```python
from build123d import *

# Parameters (mm, degrees)
SKETCH1_W           = 20
SKETCH1_H           = 155
BOSS_EXTRUDE1_DEPTH = 4
SKETCH2_W           = 20
SKETCH2_H           = 4
BOSS_EXTRUDE3_DEPTH = 50
RIB2_REACH          = 96.986
SKETCH7_WALL_W      = 290.205463948
SKETCH7_WALL_H      = 4
SKETCH8_W           = 20
SKETCH8_H           = 3
BOSS_EXTRUDE4_DEPTH = 3.5
SKETCH9_W           = 70
SKETCH9_H           = 5
BOSS_EXTRUDE6_DEPTH = 3
SKETCH10_W          = 10
SKETCH10_H          = 4
BOSS_EXTRUDE7_DEPTH = 8
SKETCH12_R          = 1.75
CUT_EXTRUDE1_DEPTH  = 10
SKETCH13_W          = 111.319070758
SKETCH13_H          = 99.743885808
CUT_EXTRUDE2_DEPTH  = 152
SKETCH14_W          = 50
SKETCH14_H          = 3
BOSS_EXTRUDE8_DEPTH = 6.5
FILLET1_R           = 1
FILLET2_R           = 2.5
SKETCH15_R          = 3.25
BOSS_EXTRUDE9_DEPTH = 3
FILLET3_R           = 10


with BuildPart() as part:
    # Sketch1 → Boss-Extrude1 (new body)
    with BuildSketch(Plane.XY):
        Rectangle(SKETCH1_W, SKETCH1_H)
    extrude(amount=BOSS_EXTRUDE1_DEPTH)

    # Sketch2 → Boss-Extrude3 (add)
    with BuildSketch(Plane.XY.offset(4)):
        with Locations((0, -75.5)):
            Rectangle(SKETCH2_W, SKETCH2_H)
    extrude(amount=BOSS_EXTRUDE3_DEPTH)

    # Sketch7 wall → Rib2 (add, up to next)
    with BuildSketch(Plane(origin=(0, -26, 16.5), x_dir=(0, 0.967074537263, -0.25449329928), z_dir=(0, 0.25449329928, 0.967074537263)), mode=Mode.PRIVATE) as rib2_sk1:
        Rectangle(SKETCH7_WALL_W, SKETCH7_WALL_H)
    rib2_tool1 = extrude(rib2_sk1.sketch, amount=-RIB2_REACH, mode=Mode.PRIVATE) - part.part
    add(rib2_tool1.solids().sort_by_distance((0, -26, 16.5))[0])

    # Sketch8 → Boss-Extrude4 (add)
    with BuildSketch(Plane.XY.offset(4)):
        with Locations((0, 76)):
            Rectangle(SKETCH8_W, SKETCH8_H)
    extrude(amount=BOSS_EXTRUDE4_DEPTH)

    # Sketch9 → Boss-Extrude6 (add)
    with BuildSketch(Plane.XY.offset(7.5)):
        with Locations((0, 77)):
            Rectangle(SKETCH9_W, SKETCH9_H)
    boss_extrude6 = extrude(amount=BOSS_EXTRUDE6_DEPTH)

    # Sketch10 → Boss-Extrude7 (add)
    with BuildSketch(Plane(origin=(0, 0, 7.5), x_dir=(-1, 0, 0), z_dir=(0, 0, -1))):
        with Locations((30, 76.5)):
            Rectangle(SKETCH10_W, SKETCH10_H)
        with Locations((-30, 76.5)):
            Rectangle(SKETCH10_W, SKETCH10_H)
    extrude(amount=BOSS_EXTRUDE7_DEPTH)

    # Sketch12 → Cut-Extrude1 (cut)
    with BuildSketch(Plane(origin=(0, 78.5, 0), x_dir=(1, 0, 0), z_dir=(0, 1, 0))):
        with Locations(Location((-31, -3, 0), (0, 0, 270))):
            Circle(SKETCH12_R)
        with Locations(Location((31, -3, 0), (0, 0, 270))):
            Circle(SKETCH12_R)
    extrude(amount=-CUT_EXTRUDE1_DEPTH, mode=Mode.SUBTRACT)

    # Sketch13 → Cut-Extrude2 (cut)
    with BuildSketch(Plane.XZ.offset(77.5)):
        with Locations((2.652852139, 20.474703111)):
            Rectangle(SKETCH13_W, SKETCH13_H)
    extrude(amount=-CUT_EXTRUDE2_DEPTH, mode=Mode.SUBTRACT)

    # Sketch14 → Boss-Extrude8 (add)
    with BuildSketch(Plane(origin=(0, 79.5, 0), x_dir=(1, 0, 0), z_dir=(0, 1, 0))):
        with Locations((0, -9)):
            Rectangle(SKETCH14_W, SKETCH14_H)
    boss_extrude8 = extrude(amount=BOSS_EXTRUDE8_DEPTH)

    # Mirror1: Boss-Extrude6, Boss-Extrude8 across plane
    add(boss_extrude6.mirror(Plane(origin=(0, 76, 0), x_dir=(0, 0, 1), z_dir=(0, -1, 0))))
    add(boss_extrude8.mirror(Plane(origin=(0, 76, 0), x_dir=(0, 0, 1), z_dir=(0, -1, 0))))

    # Fillet1
    fillet1_edges = [part.edges().sort_by_distance(p)[0] for p in [
        (30, 78.5, 7.5),
        (-30, 78.5, 7.5),
        (10, 76, 7.5),
        (-10, 76, 7.5),
        (0, 77.5, 7.5),
        (25, 76.5, 7.5),
        (-25, 76.5, 7.5),
    ]]
    fillet(fillet1_edges, radius=FILLET1_R - 0.0001)  # a hair under: the kernel refuses the full size

    # Fillet2
    fillet2_edges = [part.edges().sort_by_distance(p)[0] for p in [
        (-25, 79.5, 9),
        (25, 79.5, 9),
        (-25, 66, 9),
        (25, 66, 9),
        (-25, 72.5, 9),
        (25, 72.5, 9),
    ]]
    fillet(fillet2_edges, radius=FILLET2_R)

    # Sketch15 → Boss-Extrude9 (add)
    with BuildSketch(Plane(origin=(0, 0, 7.5), x_dir=(-1, 0, 0), z_dir=(0, 0, -1))):
        with BuildLine():
            Line((25, 86), (-25, 86))
            ThreePointArc((-25, 86), (0, 103.502), (25, 86))
        make_face()
        with Locations((0, 91.001)):
            Circle(SKETCH15_R, mode=Mode.SUBTRACT)
    extrude(amount=-BOSS_EXTRUDE9_DEPTH)

    # Fillet3
    fillet3_edges = [part.edges().sort_by_distance(p)[0] for p in [
        (-25, 86, 9),
        (25, 86, 9),
    ]]
    fillet(fillet3_edges, radius=FILLET3_R)


solid = part.part
```
The model under review builds one solid part; all positions refer to its coordinate system, in mm. A direction names the side the tool comes from. Round coordinates to 2 decimals unless told otherwise and drop trailing zeros. Order: outer loops, then holes, each group sorted by start corner. A loop starts at its lowest first (then second) coordinate and runs counter-clockwise, first axis right, second up. Notation, with made-up numbers: (48, -18.5) -> (76, -18.5) arc R25 cw to (76, 1.5) -> close; hole circle Ø8 at (48.5, -27.5). An arc over 180 degrees is marked (long way). Use a Markdown table: item, result.
Q1. We need section A-A on x = 0. Write out the cut boundary in (y, z), then the cut area to 3 significant figures.
Values:
| item | result |
|---|---|
| outline | (66, 7.5) -> (74.5, 7.5) -> (74.5, 0) -> (77.5, 0) -> (77.5, 6.5) arc R1 cw to (78.5, 7.5) -> (87.75, 7.5) -> (87.75, 10.5) -> (66, 10.5) -> close; (94.25, 7.5) -> (103.5, 7.5) -> (103.5, 10.5) -> (94.25, 10.5) -> close |
| area | 116 mm^2 |
Q2. We need section D-D on z = 9.5. Write out the cut boundary in (x, y).
Values:
| item | result |
|---|---|
| outline | (-35, 72.5) -> (-27.5, 72.5) arc R2.5 cw to (-25, 70) -> (-25, 68.5) arc R2.5 ccw to (-22.5, 66) -> (22.5, 66) arc R2.5 ccw to (25, 68.5) -> (25, 70) arc R2.5 cw to (27.5, 72.5) -> (35, 72.5) -> (35, 79.5) -> (27.5, 79.5) arc R2.5 cw to (25, 82) -> (25, 84.02) arc R10 ccw to (24.03, 88.31) arc R26.61 ccw to (-24.03, 88.31) arc R10 ccw to (-25, 84.02) -> (-25, 82) arc R2.5 cw to (-27.5, 79.5) -> (-35, 79.5) -> close; hole circle Ø6.5 at (0, 91) |
Q3. Clearance check with flat-ended pins moving along their axes: P1, Ø3.5, axis at x = -31.5, z = 9.5, coming from the +Y side; P2, Ø5, axis at x = -5, y = 79.5, coming from the -Z side; P3, Ø1.2, axis at y = 69, z = 9.5, coming from the -X side. State where each tip first meets the part, or that it passes through.
Values:
| item | result |
|---|---|
| P1 | stops at y = 79.5 |
| P2 | stops at z = 0 |
| P3 | stops at x = -25 |
Q4. We need section B-B on z = 3. Write out the cut boundary in (x, y), then the cut area to 3 significant figures.
Values:
| item | result |
|---|---|
| outline | (-35, 74.5) -> (-32.75, 74.5) -> (-32.75, 78.5) -> (-35, 78.5) -> close; (-29.25, 74.5) -> (-25, 74.5) -> (-25, 78.5) -> (-29.25, 78.5) -> close; (-10, 74.5) -> (10, 74.5) -> (10, 77.5) -> (-10, 77.5) -> close; (25, 74.5) -> (29.25, 74.5) -> (29.25, 78.5) -> (25, 78.5) -> close; (32.75, 74.5) -> (35, 74.5) -> (35, 78.5) -> (32.75, 78.5) -> close |
| area | 112 mm^2 |
Q5. Mouldability with a two-part tool opening along X and no side actions: class faces 1 (the cylindrical face through (26, 72, 9)), 2 (the flat face through (0, 81, 10.5)), 3 (the flat face through (0, 76, 0)) as +X half, -X half, draft (parallel to the pull), parting line (faces both ways), or undercut.
Values:
| item | result |
|---|---|
| face 1 | +X half |
| face 2 | draft |
| face 3 | undercut |
Q6. Tool access review of faces 4 (the flat face through (25, 83, 9)), 5 (the flat face through (0, 77.5, 3)), 6 (the flat face through (-25, 69, 9)), 7 (the flat face through (29, 78.5, 3)): name each direction out of +Z, -Z, +X, -X, +Y, -Y from which nothing blocks a thin tool from reaching the whole face with its end or side.
Values:
| item | result |
|---|---|
| face 4 | +Z, -Z, +X, +Y |
| face 5 | -Z, +Y |
| face 6 | +Z, -Z, -X, -Y |
| face 7 | -Z, +X, -X, +Y |
Q7. For line 1 (X direction, y = 77.45, z = 3); line 2 (Z direction, x = -19, y = 72); line 3 (Y direction, x = -28, z = 8), list the stretches that pass through material, from the lowest coordinate up.
Values:
| item | result |
|---|---|
| line 1 | x = -35 to -32.75, -29.25 to -25, -10 to 10, 25 to 29.25, 32.75 to 35 |
| line 2 | z = 7.5 to 10.5 |
| line 3 | y = 72.5 to 79.5 |
